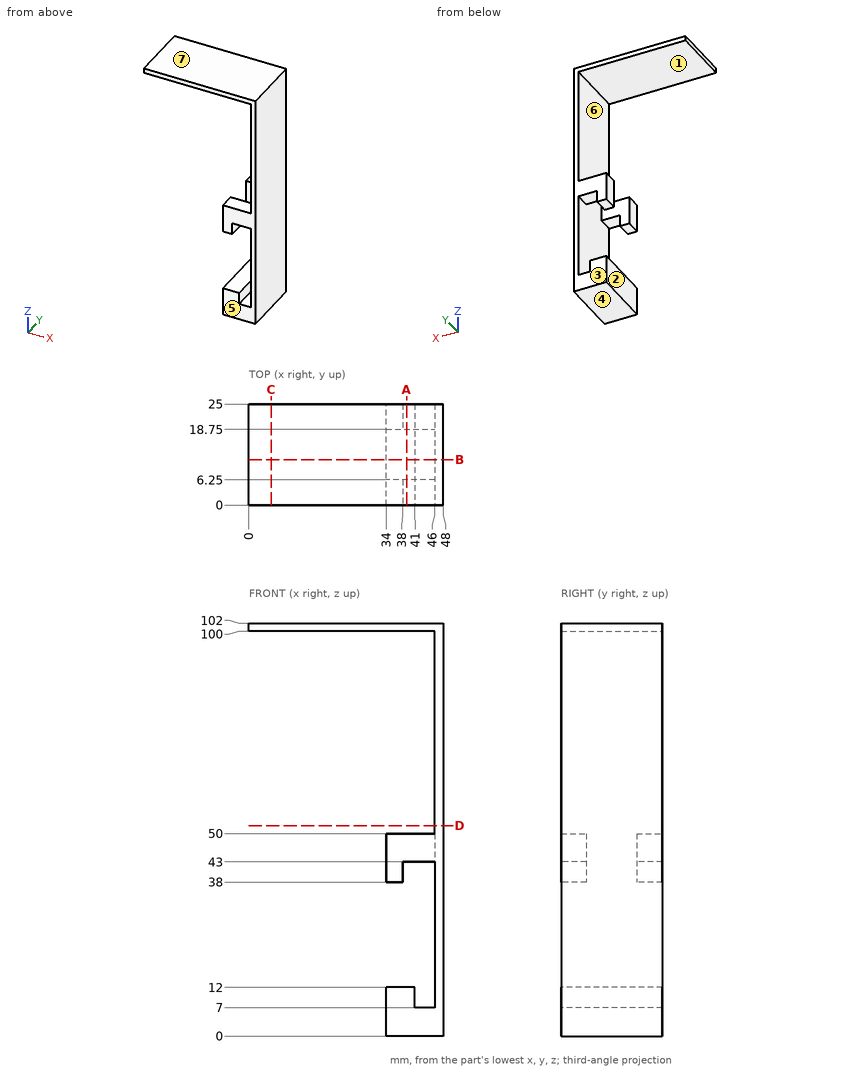
Source: three-view drawing plus pictorial views. Frame: mm from the lowest corner of the part. A direction names the side the tool comes from. Give positions to 0.01 mm unless a question says otherwise; leave off trailing zeros. Order: outer loops, then holes, each group sorted by start corner. A loop starts at its lowest first (then second) coordinate and runs counter-clockwise, first axis right, second up. Notation, with made-up numbers: M 51,9 L 73,9 A23 ccw 73,30 Z; hole C -34.5,-18.5 d5. An arc over 180 degrees is marked long. Return JSON: item names as keys, results as strings.
1) Section query B-B on y = 11.25. Output: boundary loops of the cut face in (x, z).
Taken from the geometry:
{"outline": "M 0,100 L 46,100 L 46,7 L 41,7 L 41,12 L 34,12 L 34,0 L 48,0 L 48,102 L 0,102 Z"}
2) Section query C-C on x = 5.5. Output: boundary loops of the cut face in (y, z).
Taken from the geometry:
{"outline": "M 0,100 L 25,100 L 25,102 L 0,102 Z"}
3) Access query for the marked faces 1, 2 and 3. Directions: +Z, -Z, +X, -X, +Y, -Y. A direction counts if a zero-diameter tool reaches every point of the face in a straight line with its end or side. Return the directions, or none.
Taken from the geometry:
{"face 1": "-X, +Y, -Y", "face 2": "-Z, -X, +Y, -Y", "face 3": "+Z, -Z, +X, -X, +Y"}
4) Contact query for flat-ended pins moving along their axis: pin 1 (5 mm diameter, centred on y = 22.5, z = 41.5, fed in from -X); pin 2 (6 mm diameter, centred on y = 5, z = 20.5, fed in from -X); pin 3 (12.5 mm diameter, centred on x = 21, y = 8.5, fed in from -Z). Output: stop coordinate, or through.
Taken from the geometry:
{"pin 1": "stops at x = 34", "pin 2": "stops at x = 46", "pin 3": "stops at z = 100"}
5) Mould query, pull axis Z, two halves, no side actions, for the marked faces 4, 5, 6 and 7. Classes: released by +Z, released by -Z, zero draft, split by the parting line, or undercut.
Taken from the geometry:
{"face 4": "released by -Z", "face 5": "zero draft", "face 6": "undercut", "face 7": "released by +Z"}
6) Section query A-A on x = 39. Output: boundary loops of the cut face in (y, z).
Taken from the geometry:
{"outline": "M 0,0 L 25,0 L 25,12 L 0,12 Z; M 0,43 L 6.25,43 L 6.25,50 L 0,50 Z; M 0,100 L 25,100 L 25,102 L 0,102 Z; M 18.75,43 L 25,43 L 25,50 L 18.75,50 Z"}
7) Line query: L1, parallel to X at y = 18.5, z = 8; L2, parallel to Y at x = 42.5, z = 45; L3, parallel to Z at x = 36, y = 4.5. Output: solid intervals per line, ascending. Write a range as [from, to].
Taken from the geometry:
{"L1": "x = [34, 41], [46, 48]", "L2": "y = [0, 6.25], [18.75, 25]", "L3": "z = [0, 12], [38, 50], [100, 102]"}
8) Section query D-D on z = 52. Output: boundary loops of the cut face in (x, y).
Taken from the geometry:
{"outline": "M 46,0 L 48,0 L 48,25 L 46,25 Z"}
